```python
from build123d import *

# Parameters (mm, degrees)
SKETCH_1_R          = 42.5
SKETCH_1_R_2        = 2.05
SKETCH_1_R_3        = 1.6
SKETCH_1_R_4        = 3.5
EXTRUDE_1_DEPTH     = 17
SKETCH_2_R          = 25
CUT_EXTRUDE_1_DEPTH = 10
FILLET_1_R          = 4
SKETCH_3_R          = 12
CUT_EXTRUDE_2_DEPTH = 3


with BuildPart() as part:
    # 草图1 → 凸台-拉伸1 (new body)
    with BuildSketch(Plane(origin=(0, 0, 0), x_dir=(1, 0, 0), z_dir=(0, 1, 0))):
        with Locations(Location((0, 0, 0), (0, 0, 270))):
            Circle(SKETCH_1_R)
        with Locations(Location((34, 0, 0), (0, 0, 270))):
            Circle(SKETCH_1_R_2, mode=Mode.SUBTRACT)
        with Locations(Location((29.444863729, -17, 0), (0, 0, 270))):
            Circle(SKETCH_1_R_2, mode=Mode.SUBTRACT)
        with Locations(Location((17, -29.444863729, 0), (0, 0, 270))):
            Circle(SKETCH_1_R_2, mode=Mode.SUBTRACT)
        with Locations(Location((0, -34, 0), (0, 0, 270))):
            Circle(SKETCH_1_R_2, mode=Mode.SUBTRACT)
        with Locations(Location((-17, -29.444863729, 0), (0, 0, 270))):
            Circle(SKETCH_1_R_2, mode=Mode.SUBTRACT)
        with Locations(Location((-29.444863729, -17, 0), (0, 0, 270))):
            Circle(SKETCH_1_R_2, mode=Mode.SUBTRACT)
        with Locations(Location((-34, 0, 0), (0, 0, 270))):
            Circle(SKETCH_1_R_2, mode=Mode.SUBTRACT)
        with Locations(Location((-29.444863729, 17, 0), (0, 0, 270))):
            Circle(SKETCH_1_R_2, mode=Mode.SUBTRACT)
        with Locations(Location((-17, 29.444863729, 0), (0, 0, 270))):
            Circle(SKETCH_1_R_2, mode=Mode.SUBTRACT)
        with Locations(Location((0, 34, 0), (0, 0, 270))):
            Circle(SKETCH_1_R_2, mode=Mode.SUBTRACT)
        with Locations(Location((17, 29.444863729, 0), (0, 0, 270))):
            Circle(SKETCH_1_R_2, mode=Mode.SUBTRACT)
        with Locations(Location((29.444863729, 17, 0), (0, 0, 270))):
            Circle(SKETCH_1_R_2, mode=Mode.SUBTRACT)
        with Locations(Location((7, 0, 0), (0, 0, 270))):
            Circle(SKETCH_1_R_3, mode=Mode.SUBTRACT)
        with Locations(Location((0, -7, 0), (0, 0, 270))):
            Circle(SKETCH_1_R_3, mode=Mode.SUBTRACT)
        with Locations(Location((-7, 0, 0), (0, 0, 270))):
            Circle(SKETCH_1_R_3, mode=Mode.SUBTRACT)
        with Locations(Location((0, 7, 0), (0, 0, 270))):
            Circle(SKETCH_1_R_3, mode=Mode.SUBTRACT)
        with Locations(Location((0, 0, 0), (0, 0, 270))):
            Circle(SKETCH_1_R_4, mode=Mode.SUBTRACT)
    extrude(amount=EXTRUDE_1_DEPTH)

    # 草图2 → 切除-拉伸1 (cut)
    with BuildSketch(Plane(origin=(0, 17, 0), x_dir=(1, 0, 0), z_dir=(0, 1, 0))):
        with Locations(Location((0, 0, 0), (0, 0, 270))):
            Circle(SKETCH_2_R)
    extrude(amount=-CUT_EXTRUDE_1_DEPTH, mode=Mode.SUBTRACT)

    # 圆角1
    fillet_1_edges = [part.edges().sort_by_distance(p)[0] for p in [
        (0, 7, -25),
        (0, 17, -25),
    ]]
    fillet(fillet_1_edges, radius=FILLET_1_R)

    # 草图3 → 切除-拉伸2 (cut)
    with BuildSketch(Plane.XZ):
        with Locations(Location((0, 0, 0), (0, 0, 270))):
            Circle(SKETCH_3_R)
    extrude(amount=-CUT_EXTRUDE_2_DEPTH, mode=Mode.SUBTRACT)


solid = part.part
```
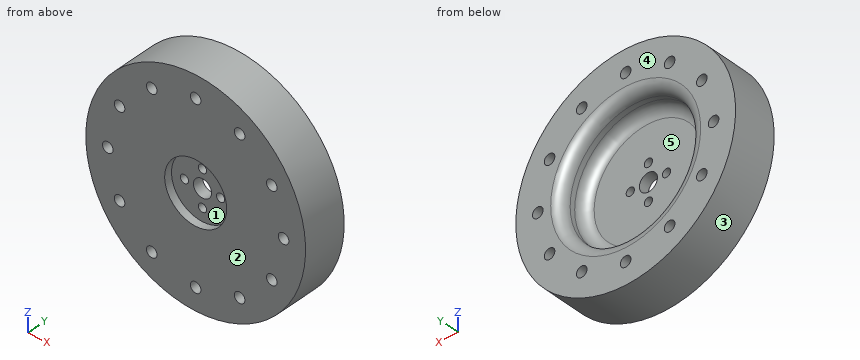
Design review of the part built by this model. Coordinates are the model's own, in mm. Face numbers are marked on the shaded views. A direction names the side the tool comes from. Give positions to 0.01 mm unless a question says otherwise; leave off trailing zeros. Write each loop counter-clockwise with the first axis right and the second up, starting at its lowest first coordinate (ties: lowest second). Pieces come first, ordered by that corner, then holes. Notation, with made-up numbers: (-26, 71) - (17, 71) arc R8 ccw to (17, 80) - close; hole circle Ø3 at (66, 40.25). An arc over 180 degrees is marked (long way). Return JSON: item names as keys, results as strings. Group by question number.
(1) Mouldability with a two-part tool opening along Z and no side actions: class the marked faces 1, 2 and 3 as +Z half, -Z half, draft (parallel to the pull), parting line (faces both ways), or undercut.
(2) We need section A-A, the plane x = 34. Give the boundary of the cut face in (y, z), then the cut area to 3 significant figures.
(3) To check wall thickness, follow probe 1 along X at (y, z) = (12.35, 0); probe 2 along X at (y, z) = (6, 0); probe 3 along Z at (x, y) = (30.5, 10.5). State the ranges of each line that lie inside material, in increasing order.
(4) Insertion check: pin 1 (4 mm diameter, centred on x = -7, z = 0, fed in from -Y); pin 2 (1 mm diameter, centred on x = -8, y = 12, fed in from -Z); pin 3 (3 mm diameter, centred on y = 3, z = -2.5, fed in from +X). Each pin has a flat end and moves straight along its axis. Give the tip position at first contact, or say it passes through.
(5) Machinability: for the marked faces 4 and 5, which of the approach directions +Z, -Z, +X, -X, +Y, -Y give a long, thin tool a straight path to every point of the face, cutting with its end or side? Answer none if there is none.
(6) We need section B-B, the plane y = 1.75. Give the number of separate pieces and of enclosed holes in the cut face, then the cut area to 3 significant figures.
Reported:
{
 "1": {"face 1": "undercut", "face 2": "draft", "face 3": "parting line"},
 "2": {"outline": "(0, -25.5) - (17, -25.5) - (17, -2.05) - (0, -2.05) - close; (0, 2.05) - (17, 2.05) - (17, 25.5) - (0, 25.5) - close", "area": "797 mm2"},
 "3": {"probe 1": "x = -42.5 to -36.05, -31.95 to -25, 25 to 31.95, 36.05 to 42.5", "probe 2": "x = -42.5 to -36.05, -31.95 to -8.6, -5.4 to -3.5, 3.5 to 5.4, 8.6 to 31.95, 36.05 to 42.5", "probe 3": "z = -29.6 to -18.76, -15.24 to 15.24, 18.76 to 29.6"},
 "4": {"pin 1": "stops at y = 3", "pin 2": "stops at z = -41.83", "pin 3": "stops at x = 42.49"},
 "5": {"face 4": "+Z, -Z, +X, -X, +Y", "face 5": "+Y"},
 "6": {"separate pieces": "1", "enclosed holes": "13", "area": "5,060 mm2"}
}
